The listing builds one solid part. Answer for the finished solid, in the listing's coordinates (mm). Face numbers are marked on the shaded views. A direction names the side the tool comes from. Give positions to 0.01 mm unless a question says otherwise; leave off trailing zeros. Loops run counter-clockwise (first coordinate to the right, second up) from the corner with the lowest first, then second, coordinate; pieces in that order, holes last.
Item 1: A tool of negligible diameter and unlimited length cuts with its end or side. For the marked faces 4, 5 and 6, from which of +Z, -Z, +X, -X, +Y, -Y can it reach the whole face along a straight path? Write none if from no direction.
Item 2: Section B-B, the plane z = 132.5 is taken. Give the vertices of the cut face in (x, y).
Item 3: Section D-D, the plane x = 62.5 is taken. Give the vertices of the cut face in (y, z), and give its area (3 significant figures).
Item 4: Each of these flat-tipped pins is pushed along its axis until it touches: pin 1 Ø6 at (x, y) = (121, 4) entering from -Z; pin 2 Ø10 at (x, y) = (106.5, 10) entering from +Z; pin 3 Ø19 at (x, z) = (3.23, 158.8) entering from +Y; pin 4 Ø2 at (x, y) = (-92.5, 7.5) entering from -Z. Where does it stop, or does it pass through?
Item 5: The mould has two halves that part along Z. Classify the marked faces 1, 2 and 3: pulls with the +Z half, pulls with the -Z half, needs draft (parallel to the pull), parting line crosses it, or undercut.
Item 6: Consider line 1 along X through (y, z) = (14.5, 63); line 2 along X through (y, z) = (10.5, 105); line 3 along Z through (x, y) = (1, 3.25). Determine where each line is inside the solid, lowest interval first.
Item 7: Section A-A, the plane x = 101 is taken. Give the vertices of the cut face in (y, z), and give its area (3 significant figures).
Item 8: Section C-C, the plane y = 16.25 is taken. Give the vertices of the cut face in (x, z).
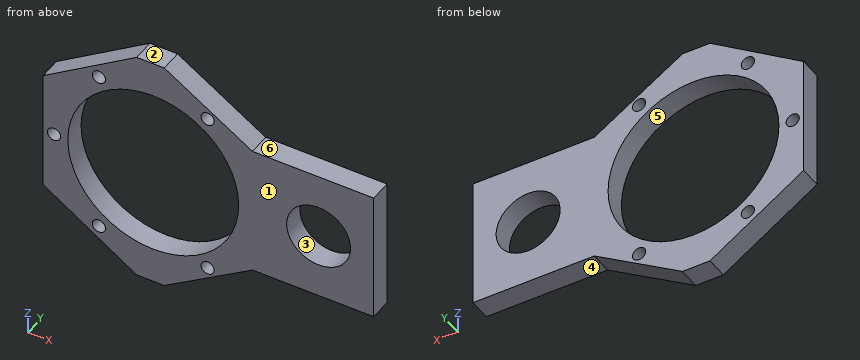
Solid Edge part; units mm, degrees
sketch "Sketch1" plane through (0, 0, 0) normal (0, -1, 0) x (1, 0, 0)
  line L0 (-146.0885, -26.4817) -> (153.9115, -26.4817)
  line L1 (153.9115, -26.4817) -> (153.9115, 193.5183)
  line L2 (-146.0885, 193.5183) -> (153.9115, 193.5183)
  line L3 (-146.0885, -26.4817) -> (-146.0885, 193.5183)
  dimension "D1" = 146.0885
  dimension "D2" = 153.9115
extrude "Protrusion1" add sketch "Sketch1" against normal blind 20
sketch "Sketch2" plane through (3.9115, 20, 48.5183) normal (0, 1, 0) x (-1, 0, 0)
  circle A0 centre (50, 35) radius 77.5
extrude "Cutout1" cut sketch "Sketch2" against normal through all
sketch "Sketch3" plane through (3.9115, 20, 38.5183) normal (0, 1, 0) x (-1, 0, 0)
  circle A0 centre (-100, 45) radius 29
  dimension "D1" = 100
extrude "Cutout2" cut sketch "Sketch3" against normal through all
sketch "Sketch4" plane through (3.9115, 20, 73.5183) normal (0, 1, 0) x (-1, 0, 0)
  line L0 (150, 65) -> (65, 120)
  line L1 (65, 120) -> (150, 120)
  line L2 (150, 120) -> (150, 65)
  line L3 (-150, 120) -> (-150, 70)
  line L4 (-40, 70) -> (-150, 70)
  line L5 (40, 120) -> (-40, 70)
  line L6 (-150, 120) -> (40, 120)
  dimension "D1" = 150
  dimension "D2" = 150
  dimension "D3" = 65
  dimension "D4" = 150
  dimension "D5" = 40
  dimension "D6" = 150
extrude "Cutout3" cut sketch "Sketch4" against normal through all
hole "Hole1" at (-136.0885, 20, 83.5183) direction (0, -1, 0) diameter 12 end up to next
hole "Hole2" at (-95.4086, 20, 8.2354) direction (0, -1, 0) diameter 12 end up to next
hole "Hole3" at (3.2316, 20, 8.2354) direction (0, -1, 0) diameter 12 end up to next
mirror "Mirror1" about plane through (-73.5885, 5, 83.5183) normal (0, 0, 1) of "Cutout3", "Hole1", "Hole2", "Hole3"
Worked answers:
1. face 4: -Z, +X, +Y, -Y
1. face 5: +Y, -Y
1. face 6: +Z, +X, +Y, -Y
2. outline: (-146.09, 0) - (-106.15, 0) - (-106.15, 20) - (-146.09, 20) - close; (13.97, 0) - (153.91, 0) - (153.91, 20) - (13.97, 20) - close
3. outline: (0, 23.52) - (20, 23.52) - (20, 143.52) - (0, 143.52) - close
3. area: 2,400 mm2
4. pin 1: stops at z = 23.52
4. pin 2: stops at z = 143.52
4. pin 3: stops at y = 20
4. pin 4: stops at z = -6.8
5. face 1: needs draft
5. face 2: pulls with the +Z half
5. face 3: undercut
6. line 1: x = -146.09 to -120.82, 28.65 to 83.42, 124.41 to 153.91
6. line 2: x = -146.09 to -120.55, 28.37 to 84.43, 123.39 to 153.91
6. line 3: z = -3.3 to 2.67, 13.8 to 21.96, 145.07 to 153.23, 164.37 to 170.34
7. outline: (0, 23.52) - (20, 23.52) - (20, 54.66) - (0, 54.66) - close; (0, 112.37) - (20, 112.37) - (20, 143.52) - (0, 143.52) - close
7. area: 1,250 mm2
8. outline: (-146.09, 28.52) - (-61.09, -26.48) - (-36.09, -26.48) - (43.91, 23.52) - (153.91, 23.52) - (153.91, 143.52) - (43.91, 143.52) - (-36.09, 193.52) - (-61.09, 193.52) - (-146.09, 138.52) - close; hole circle Ø12 at (-136.09, 83.52); hole circle Ø155 at (-46.09, 83.52); hole circle Ø12 at (-95.41, 8.24); hole circle Ø12 at (-95.41, 158.8); hole circle Ø12 at (3.23, 8.24); hole circle Ø12 at (3.23, 158.8); hole circle Ø58 at (103.91, 83.52)
